The listing builds one solid part. Answer for the finished solid, in the listing's coordinates (mm). Face numbers are marked on the shaded views. A direction names the side the tool comes from. Round coordinates to 2 decimals unless told otherwise and drop trailing zeros. Write each loop counter-clockwise with the first axis right and the second up, starting at its lowest first coordinate (ties: lowest second). Pieces come first, ordered by that corner, then holes. Notation, with made-up numbers: (53.25, -5) - (74.25, -5) arc R20 cw to (74.25, 7) - close; hole circle Ø11 at (16.25, -29.5). An arc over 180 degrees is marked (long way). Return JSON: item names as keys, results as strings. Group by question number.
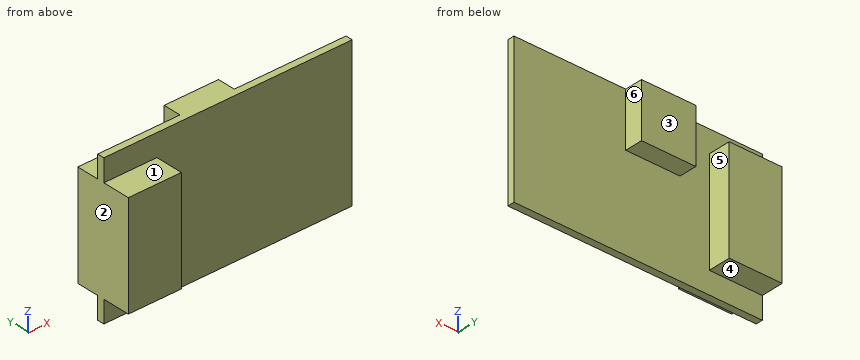
from build123d import *

# Parameters (mm, degrees)
SKETCH1_W           = 24.384
SKETCH1_H           = 14.5
BOSS_EXTRUDE1_DEPTH = 0.6858
SKETCH2_W           = 5.207
SKETCH2_H           = 10.16
BOSS_EXTRUDE2_DEPTH = 2.2098
SKETCH3_W           = 5.207
SKETCH3_H           = 10.16
BOSS_EXTRUDE3_DEPTH = 2.7178
SKETCH4_W           = 5.334
SKETCH4_H           = 5.334
BOSS_EXTRUDE4_DEPTH = 1.7526


with BuildPart() as part:
    # Sketch1 → Boss-Extrude1 (new body)
    with BuildSketch(Plane(origin=(0, 0, 0), x_dir=(1, 0, 0), z_dir=(0, 1, 0))):
        with Locations((12.192, 7.25)):
            Rectangle(SKETCH1_W, SKETCH1_H)
    extrude(amount=BOSS_EXTRUDE1_DEPTH)

    # Sketch2 → Boss-Extrude2 (add)
    with BuildSketch(Plane(origin=(0, 0.6858, 0), x_dir=(1, 0, 0), z_dir=(0, 1, 0))):
        with Locations((2.6035, 7.261)):
            Rectangle(SKETCH2_W, SKETCH2_H)
    extrude(amount=BOSS_EXTRUDE2_DEPTH)

    # Sketch3 → Boss-Extrude3 (add)
    with BuildSketch(Plane.XZ):
        with Locations((2.6035, -7.261)):
            Rectangle(SKETCH3_W, SKETCH3_H)
    extrude(amount=BOSS_EXTRUDE3_DEPTH)

    # Sketch4 → Boss-Extrude4 (add)
    with BuildSketch(Plane(origin=(0, 0.6858, 0), x_dir=(1, 0, 0), z_dir=(0, 1, 0))):
        with Locations((10.7442, 2.667)):
            Rectangle(SKETCH4_W, SKETCH4_H)
    extrude(amount=BOSS_EXTRUDE4_DEPTH)


solid = part.part
(1) Find section A-A (y = 1.5). Write down the section's boundary in (x, z).
(2) Consider line 1 (X direction, y = 0.95, z = -2.25); line 2 (Y direction, x = 10.5, z = -9); line 3 (X direction, y = -2.25, z = -8.25). Determine where each line is inside the solid, lowest interval first.
(3) Flat-ended cylindrical pins translate along their axes: pin 1 (6 mm diameter, centred on x = 14.5, z = -3.5, fed in from +Y); pin 2 (0.5 mm diameter, centred on x = 11, y = 1.5, fed in from -Z); pin 3 (0.7 mm diameter, centred on y = 1.5, z = -5, fed in from +X). Find the tip coordinate at first contact, or state that the pin passes through.
(4) Find section B-B (z = -10.25). Write down the section's boundary in (x, y), plus the area to 3 significant figures.
(5) Find section D-D (z = -2.75). Write down the section's boundary in (x, y).
(6) Determine the mould class of the marked faces 4, 5 and 6 for opening direction X: +X half, -X half, draft (parallel to the pull), parting line (faces both ways), or undercut.
(7) For the marked faces 1, 2 and 3, determine the directions among +Z, -Z, +X, -X, +Y, -Y from which every point of the face is accessible in a straight line to the end or side of a thin tool.
(8) Find section C-C (x = 3.25). Write down the section's boundary in (y, z), plus the area to 3 significant figures.
Check sheet entries:
{
 "1": {"outline": "(0, -12.34) - (5.21, -12.34) - (5.21, -2.18) - (0, -2.18) - close; (8.08, -5.33) - (13.41, -5.33) - (13.41, 0) - (8.08, 0) - close"},
 "2": {"line 1": "x = 0 to 5.21, 8.08 to 13.41", "line 2": "y = 0 to 0.69", "line 3": "x = 0 to 5.21"},
 "3": {"pin 1": "stops at y = 2.44", "pin 2": "stops at z = -5.33", "pin 3": "stops at x = 13.41"},
 "4": {"outline": "(0, -2.72) - (5.21, -2.72) - (5.21, 0) - (24.38, 0) - (24.38, 0.69) - (5.21, 0.69) - (5.21, 2.9) - (0, 2.9) - close", "area": "42.4 mm^2"},
 "5": {"outline": "(0, -2.72) - (5.21, -2.72) - (5.21, 0) - (24.38, 0) - (24.38, 0.69) - (13.41, 0.69) - (13.41, 2.44) - (8.08, 2.44) - (8.08, 0.69) - (5.21, 0.69) - (5.21, 2.9) - (0, 2.9) - close"},
 "6": {"face 4": "draft", "face 5": "undercut", "face 6": "+X half"},
 "7": {"face 1": "+Z, +X, -X, -Y", "face 2": "+Z, -Z, -X, +Y, -Y", "face 3": "+Z, -Z, +X, +Y"},
 "8": {"outline": "(-2.72, -12.34) - (0, -12.34) - (0, -14.5) - (0.69, -14.5) - (0.69, -12.34) - (2.9, -12.34) - (2.9, -2.18) - (0.69, -2.18) - (0.69, 0) - (0, 0) - (0, -2.18) - (-2.72, -2.18) - close", "area": "60.0 mm^2"}
}
